Check sheet for the modelled part. Datum: model origin and axes. Units: mm. Face numbers are marked on the shaded views. Give positions to 0.01 mm unless a question says otherwise; leave off trailing zeros. Order: outer loops, then holes, each group sorted by start corner. A loop starts at its lowest first (then second) coordinate and runs counter-clockwise, first axis right, second up.
Autodesk Inventor part; units mm, degrees
ref_plane "YZ Plane" through (0, 0, 0) normal (1, 0, 0) x (0, 1, 0)
ref_plane "XZ Plane" through (0, 0, 0) normal (0, 1, 0) x (-1, 0, 0)
ref_plane "XY Plane" through (0, 0, 0) normal (0, 0, 1) x (1, 0, 0)
sketch "Sketch1" plane through (0, 0, 0) normal (0, 0, 1) x (1, 0, 0)
  line L0 (-18.5, 15.25) -> (18.5, 15.25)
  line L1 (18.5, 15.25) -> (18.5, -15.25)
  line L2 (18.5, -15.25) -> (-18.5, -15.25)
  line L3 (-18.5, -15.25) -> (-18.5, 15.25)
  point P0 (0, 0)
  point P1 (0, 15.25)
  point P2 (18.5, 0)
  dimension "d0" = 37
  dimension "d1" = 30.5
extrude "Extrusion1" add sketch "Sketch1" along normal blind 15
sketch "Sketch2" plane through (0, 0, 15) normal (0, 0, 1) x (1, 0, 0)
  circle A0 centre (14.605, 0) radius 1.65
  circle A1 centre (-14.605, 0) radius 1.65
  line L0 (14.605, 0) -> (-14.605, 0) construction
  point P0 (0, 0)
  point P1 (0, 0)
  dimension "d4" = 3.3
  dimension "d5" = 3.3
  dimension "d6" = 29.21
extrude "Extrusion2" cut sketch "Sketch2" against normal up to next
properties part number "bigeasydriver"
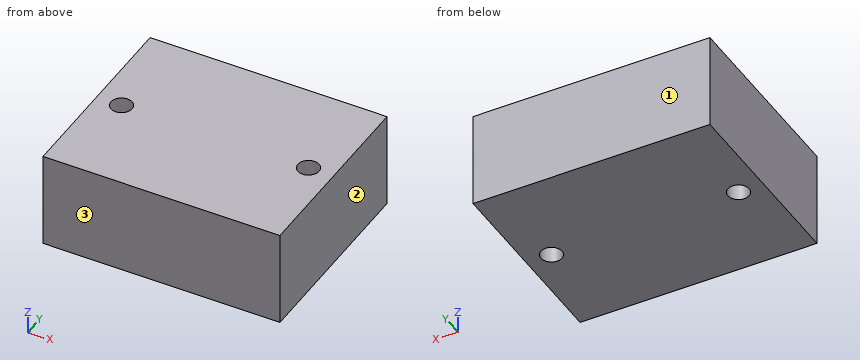
(1) Cross-section at A-A on y = 0. Enter the section's corners in (x, z) (3 decimals), then the cut area to 3 significant figures.
Response values:
outline: (-18.5, 0) - (-16.255, 0) - (-16.255, 15) - (-18.5, 15) - close; (-12.955, 0) - (12.955, 0) - (12.955, 15) - (-12.955, 15) - close; (16.255, 0) - (18.5, 0) - (18.5, 15) - (16.255, 15) - close
area: 456 mm2
(2) Material ranges on L1, parallel to Y at x = -14.5, z = 7.5; L2, parallel to X at y = 1, z = 4; L3, parallel to X at y = -1.5, z = 5, recorded low to high.
Response values:
L1: y = -15.25 to -1.65, 1.65 to 15.25
L2: x = -18.5 to -15.92, -13.29 to 13.29, 15.92 to 18.5
L3: x = -18.5 to -15.29, -13.92 to 13.92, 15.29 to 18.5
(3) Release check for a two-part mould opening along Y. For the marked faces 1, 2 and 3 record: released by +Y, released by -Y, zero draft, split by the parting line, or undercut.
Response values:
face 1: released by +Y
face 2: zero draft
face 3: released by -Y
